from build123d import *

# Parameters (mm, degrees)
F1_DEPTH = 10
F3_DEPTH = 10
F5_DEPTH = 5


with BuildPart() as f1:
    # F0 (on Front) → F1 (new body)
    with BuildSketch(Plane.XZ):
        with BuildLine():
            Line((-25, 75), (-25, 0))
            Line((-25, 0), (25, 0))
            Line((25, 0), (25, 75))
            Line((25, 75), (10, 75))
            Line((10, 75), (10, 50))
            ThreePointArc((10, 50), (0, 40), (-10, 50))
            Line((-10, 50), (-10, 75))
            Line((-10, 75), (-25, 75))
        make_face()
    extrude(amount=F1_DEPTH)

    # F2 (on Top) → F3 (join)
    with BuildSketch(Plane.XY):
        with BuildLine():
            Line((10, -10), (-10, -10))
            Line((-10, -10), (-25, -10))
            Line((-25, -10), (-25, -25))
            ThreePointArc((-25, -25), (0, -50), (25, -25))
            Line((25, -25), (25, -10))
            Line((25, -10), (10, -10))
        make_face()
    extrude(amount=F3_DEPTH)

    # F4 (on face) → F5 (cut)
    with BuildSketch(Plane.YZ.offset(25)):
        Polygon((0, 20), (-10, 20), (-10, 10), (-15, 10), (-15, 0), (0, 0), align=None)
    extrude(amount=-F5_DEPTH, mode=Mode.SUBTRACT)


solid = f1.part
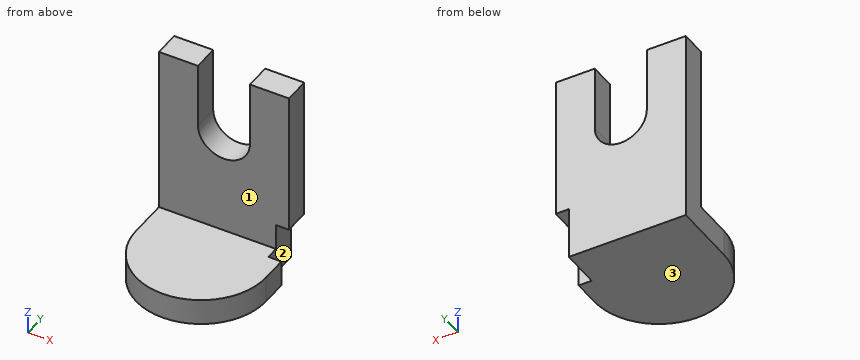
Source: CAD feature listing. Evaluate the final solid. Frame: model axes, mm. Face numbers are marked on the shaded views. A direction names the side the tool comes from. Give positions to 0.01 mm unless a question says otherwise; leave off trailing zeros. Loops run counter-clockwise (first coordinate to the right, second up) from the corner with the lowest first, then second, coordinate; pieces in that order, holes last. Notation, with made-up numbers: (25.25, 75.5) -> (60.25, 75.5) arc R29 ccw to (60.25, 107.5) -> close; hole circle Ø11 at (54.25, 24). An arc over 180 degrees is marked (long way). Use a Markdown table: item, result. Add a question column.
1) Reachability of the marked faces 1, 2 and 3 from +Z, -Z, +X, -X, +Y, -Y: full face, straight path, thin tool, end or side. Return the list, or none.
2) Section query C-C, the plane x = 0. Return the cut outline in (y, z).
3) Section query B-B, the plane z = 70.5. Return the cut outline in (x, y).
4) Section query A-A, the plane y = -8.5. Return the cut outline in (x, z), then the cut area to 3 significant figures.
5) Line query: line 1 along X through (y, z) = (-7.5, 56.5); line 2 along Z through (x, y) = (-7, -45.5); line 3 along Y through (x, z) = (-21, 67). Output: solid intervals per line, ascending. Write a range as [from, to].
6) First-contact query: pin 1 (8 mm diameter, centred on x = -2, y = -11.5, fed in from +Z); pin 2 (12 mm diameter, centred on x = -8.5, y = -28.5, fed in from +Z); pin 3 (4.5 mm diameter, centred on y = -7, z = 6.5, fed in from +X). Flat tips, straight axial feed; report the tip coordinate or a pass-through.
7) Section query D-D, the plane z = 11. Return the cut outline in (x, y), then the cut area to 3 significant figures.
Numbers:
| question | item | result |
|---|---|---|
| 1 | face 1 | +Z, +X, -X, -Y |
| 1 | face 2 | -Z, +X, +Y |
| 1 | face 3 | -Z, +X, -X, +Y, -Y |
| 2 | outline | (-50, 0) -> (0, 0) -> (0, 40) -> (-10, 40) -> (-10, 10) -> (-50, 10) -> close |
| 3 | outline | (-25, -10) -> (-10, -10) -> (-10, 0) -> (-25, 0) -> close; (10, -10) -> (25, -10) -> (25, 0) -> (10, 0) -> close |
| 4 | outline | (-25, 0) -> (20, 0) -> (20, 20) -> (25, 20) -> (25, 75) -> (10, 75) -> (10, 50) arc R10 cw to (-10, 50) -> (-10, 75) -> (-25, 75) -> close |
| 4 | area | 2,990 mm2 |
| 5 | line 1 | x = [-25, -10], [10, 25] |
| 5 | line 2 | z = [0, 10] |
| 5 | line 3 | y = [-10, 0] |
| 6 | pin 1 | stops at z = 41.79 |
| 6 | pin 2 | stops at z = 10 |
| 6 | pin 3 | stops at x = 20 |
| 7 | outline | (-25, -10) -> (20, -10) -> (20, 0) -> (-25, 0) -> close |
| 7 | area | 450 mm2 |
